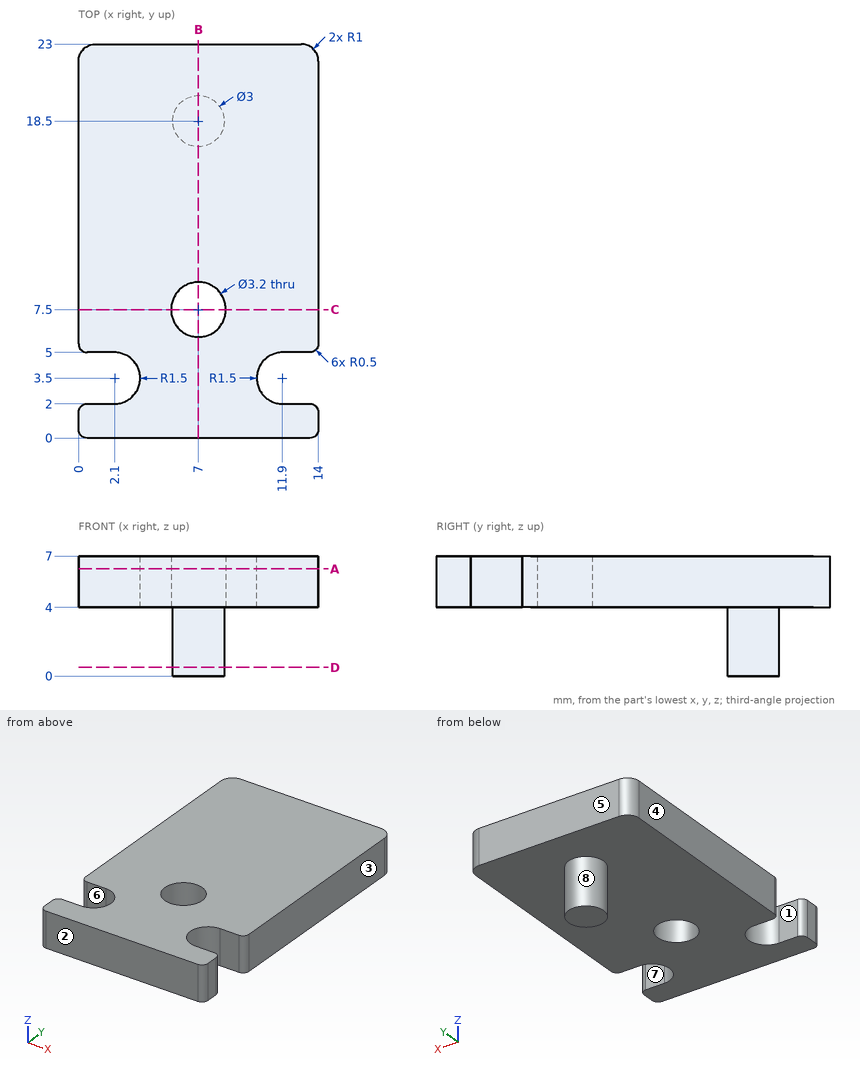
Could you check a few things on this drawing? It's one solid part, dimensions in mm from its lowest x, y, z. A direction names the side the tool comes from. Give positions to 0.01 mm unless a question says otherwise; leave off trailing zeros. Order: outer loops, then holes, each group sorted by start corner. A loop starts at its lowest first (then second) coordinate and runs counter-clockwise, first axis right, second up.
1. Suppose I cut it at B-B (x = 7). Write out the boundary of the cut face in (y, z).
Answers below:
outline: (0, 4) - (5.9, 4) - (5.9, 7) - (0, 7) - close; (9.1, 4) - (17, 4) - (17, 0) - (20, 0) - (20, 4) - (23, 4) - (23, 7) - (9.1, 7) - close
2. Thinking about a two-plate mould opening in Y: for the marked faces 1, 2 and 3, which applies, +Y half, -Y half, draft (parallel to the pull), parting line (faces both ways), or undercut?
Answers below:
face 1: undercut
face 2: -Y half
face 3: draft
3. I need wall thicknesses on L1, parallel to Y at x = 7, z = 5.75; L2, parallel to Z at x = 1, y = 8.25; L3, parallel to Y at x = 6, z = 1. Which ranges of each line are inside material? Lowest first, please.
Answers below:
L1: y = 0 to 5.9, 9.1 to 23
L2: z = 4 to 7
L3: y = 17.38 to 19.62
4. Which directions (+Z, -Z, +X, -X, +Y, -Y) give clear straight access to the entire face, cutting with the end or side of a thin tool? Please do the marked faces 4, 5, 6, 7 and 8.
Answers below:
face 4: +Z, -Z, -X, +Y, -Y
face 5: +Z, -Z, +X, -X, +Y
face 6: +Z, -Z, -X
face 7: +Z, -Z, +X
face 8: -Z
5. Suppose I cut it at A-A (z = 6.25). Write out the boundary of the cut face in (x, y).
Answers below:
outline: (0, 0.5) arc R0.5 ccw to (0.5, 0) - (13.5, 0) arc R0.5 ccw to (14, 0.5) - (14, 1.5) arc R0.5 ccw to (13.5, 2) - (11.9, 2) arc R1.5 cw to (11.9, 5) - (13.5, 5) arc R0.5 ccw to (14, 5.5) - (14, 22) arc R1 ccw to (13, 23) - (1, 23) arc R1 ccw to (0, 22) - (0, 5.5) arc R0.5 ccw to (0.5, 5) - (2.1, 5) arc R1.5 cw to (2.1, 2) - (0.5, 2) arc R0.5 ccw to (0, 1.5) - close; hole circle Ø3.2 at (7, 7.5)
6. Suppose I cut it at D-D (z = 0.5). Write out the boundary of the cut face in (x, y), plus the area to 3 significant figures.
Answers below:
outline: circle Ø3 at (7, 18.5)
area: 7.07 mm2
7. Suppose I cut it at C-C (y = 7.5). Write out the boundary of the cut face in (x, z).
Answers below:
outline: (0, 4) - (5.4, 4) - (5.4, 7) - (0, 7) - close; (8.6, 4) - (14, 4) - (14, 7) - (8.6, 7) - close
8. For pin 1 (1 mm diameter, centred on x = 5, y = 6.5, fed in from -Z); pin 2 (0.5 mm diameter, centred on x = 13, z = 5.5, fed in from -Y), each with a flat end and sliding along its axis, tell me the tip position at first contact or that it passes through.
Answers below:
pin 1: stops at z = 4
pin 2: stops at y = 0
